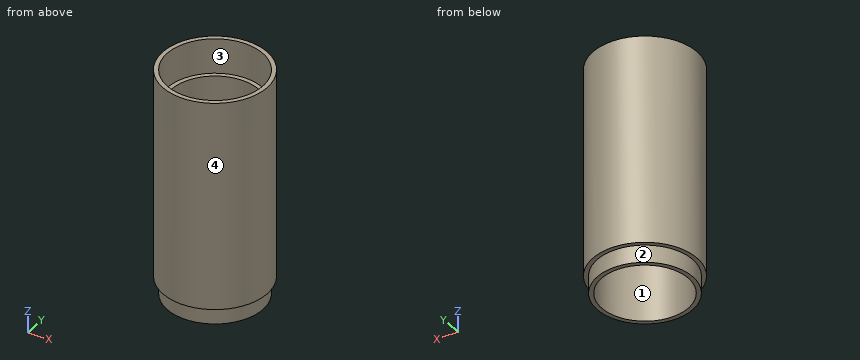
```python
from build123d import *

# Parameters (mm, degrees)
SKETCH_2_R          = 60
EXTRUDE_1_DEPTH     = 200
SKETCH_3_R          = 50
CUT_EXTRUDE_1_DEPTH = 200
EXTRUDE_START       = 20
SKETCH_4_R          = 55
SKETCH_4_R_2        = 50
EXTRUDE_2_DEPTH     = 20
SKETCH_5_R          = 60
SKETCH_5_R_2        = 55
EXTRUDE_3_DEPTH     = 40


with BuildPart() as part:
    # 草图2 → 凸台-拉伸1 (new body)
    with BuildSketch(Plane.XY):
        with Locations((-112.606133367, 79.56790028)):
            Circle(SKETCH_2_R)
    extrude(amount=EXTRUDE_1_DEPTH)

    # 草图3 → 切除-拉伸1 (cut)
    with BuildSketch(Plane(origin=(0, 0, 0), x_dir=(-1, 0, 0), z_dir=(0, 0, -1))):
        with Locations((112.606133367, 79.56790028)):
            Circle(SKETCH_3_R)
    extrude(amount=-CUT_EXTRUDE_1_DEPTH, mode=Mode.SUBTRACT)

    # 草图4 → 凸台-拉伸2 (add)
    with BuildSketch(Plane(origin=(0, 0, 0), x_dir=(-1, 0, 0), z_dir=(0, 0, -1)).offset(EXTRUDE_START)):
        with Locations((112.606133367, 79.56790028)):
            Circle(SKETCH_4_R)
        with Locations((112.606133367, 79.56790028)):
            Circle(SKETCH_4_R_2, mode=Mode.SUBTRACT)
    extrude(amount=-EXTRUDE_2_DEPTH)

    # 草图5 → 凸台-拉伸3 (add)
    with BuildSketch(Plane.XY.offset(200)):
        with Locations((-112.606133367, 79.56790028)):
            Circle(SKETCH_5_R)
        with Locations(Location((-112.606133367, 79.56790028, 0), (0, 0, 180))):
            Circle(SKETCH_5_R_2, mode=Mode.SUBTRACT)
    extrude(amount=EXTRUDE_3_DEPTH)


solid = part.part
```
Read the model definition and answer for the solid it produces. Units are mm, in the model's axes. Face numbers are marked on the shaded views. A direction names the side the tool comes from. Coordinates: 2 decimals unless noted, no trailing zeros. Write each loop counter-clockwise with the first axis right and the second up, starting at its lowest first coordinate (ties: lowest second). Pieces come first, ordered by that corner, then holes. Notation, with made-up numbers: (66, 0) - (86, 0) arc R19 ccw to (86, 9) - close; hole circle Ø1 at (86.5, 61). An arc over 180 degrees is marked (long way). Answer as a JSON object with one key per item and string values. Group by question number.
1. Consider L1, parallel to Y at x = -114.5, z = 150; L2, parallel to X at y = 76.5, z = 21.5; L3, parallel to X at y = 95.5, z = 163.5. Determine where each line is inside the solid, lowest interval first. Write a range as [from, to].
2. The mould has two halves that part along X. Classify the marked faces 3 and 4: +X half, -X half, draft (parallel to the pull), parting line (faces both ways), or undercut.
3. A cutting plane is placed at A-A (y = 75). Determine the outline of the cut face in (x, z), plus the area to 3 significant figures.
4. Which of the six approach directions +Z, -Z, +X, -X, +Y, -Y give full straight-line access (tool end or side, diameter ignored) to the marked faces 1 and 2?
5. A cutting plane is placed at B-B (x = -159). Determine the outline of the cut face in (y, z), plus the area to 3 significant figures.
6. A cutting plane is placed at C-C (z = 19). Determine the outline of the cut face in (x, y).
7. Each of these flat-tipped pins is pushed along its axis until it touches: P1, Ø8, axis at x = -111.5, z = 101.5, coming from the -Y side; P2, Ø3, axis at x = -74, z = 179, coming from the +Y side; P3, Ø1, axis at x = -106.5, z = 158.5, coming from the -Y side. Where does it stop, or does it pass through?
Worked out:
{
 "1": {"L1": "y = [19.6, 29.6], [129.53, 139.54]", "L2": "x = [-172.53, -162.51], [-62.7, -52.68]", "L3": "x = [-170.45, -160], [-65.21, -54.76]"},
 "2": {"face 3": "undercut", "face 4": "parting line"},
 "3": {"outline": "(-172.43, 0) - (-167.42, 0) - (-167.42, -20) - (-162.4, -20) - (-162.4, 200) - (-167.42, 200) - (-167.42, 240) - (-172.43, 240) - close; (-62.82, -20) - (-57.8, -20) - (-57.8, 0) - (-52.78, 0) - (-52.78, 240) - (-57.8, 240) - (-57.8, 200) - (-62.82, 200) - close", "area": "4,620 mm²"},
 "4": {"face 1": "+Z, -Z", "face 2": "-Z"},
 "5": {"outline": "(41.52, 0) - (50.03, 0) - (50.03, -20) - (60.92, -20) - (60.92, 200) - (50.03, 200) - (50.03, 240) - (41.52, 240) - close; (98.21, -20) - (109.11, -20) - (109.11, 0) - (117.62, 0) - (117.62, 240) - (109.11, 240) - (109.11, 200) - (98.21, 200) - close", "area": "8,880 mm²"},
 "6": {"outline": "circle Ø120 at (-112.61, 79.57); hole circle Ø100 at (-112.61, 79.57)"},
 "7": {"P1": "stops at y = 19.57", "P2": "stops at y = 126.72", "P3": "stops at y = 19.83"}
}
